CAD build for the part. Positions are in the model's coordinates, mm. A direction names the side the tool comes from. Coordinates: 2 decimals unless noted, no trailing zeros. Loops run counter-clockwise (first coordinate to the right, second up) from the corner with the lowest first, then second, coordinate; pieces in that order, holes last.
1) Saw through at C-C, the plane x = 15.3. Write the cut outline in (y, z).
2) Wall check: line 1 along Y through (x, z) = (0, 2.45); line 2 along Z through (x, y) = (3, 0.5). Give the ranges that are in metal, low to high.
3) Saw through at D-D, the plane y = -1.5. Write the cut outline in (x, z).
4) Saw through at A-A, the plane x = 0. Write the cut outline in (y, z).
5) Pin check, flat tips, straight feed: pin 1 Ø3.5 at (x, y) = (8, -0.5) entering from +Z; pin 2 Ø3 at (y, z) = (-3, 4.5) entering from +X; pin 3 Ø0.7 at (x, y) = (15.3, 0) entering from -Z; pin 4 Ø4 at (x, y) = (0, 0) entering from -Z. Stop position of each tip, or through.
6) Which spindle directions (+Z, -Z, +X, -X, +Y, -Y) get a long thin tool onto all of the face, cutting with end or side? Do faces 1 (the cylindrical face through (18.354, 0.23, 0.986)), 2 (the cylindrical face through (0.509, 2.294, 4.218)), 3 (the flat face through (-1, 1, 2.1)). Say none if no direction does.
7) Saw through at B-B, the plane z = 3.95. Write the cut outline in (x, y).
Autodesk Fusion 360 part; units mm, degrees
sketch "スケッチ1" plane through (0, 0, 0) normal (0, 0, 1) x (1, 0, 0)
  line L0 (2.1071, 3.4) -> (-2.1071, 3.4) construction
  line L1 (-2.1071, -3.4) -> (2.1071, -3.4) construction
  line L2 (22.8, 3.4) -> (-22.8, 3.4) construction
  line L3 (-22.8, 3.4) -> (-22.8, -3.4) construction
  line L4 (-22.8, -3.4) -> (22.8, -3.4) construction
  line L5 (22.8, -3.4) -> (22.8, 3.4) construction
  line L6 (22.8, 3.4) -> (-22.8, -3.4) construction
  line L7 (-22.8, 3.4) -> (22.8, -3.4) construction
  line L8 (-2.1071, 3.4) -> (-20.4231, 2.497)
  line L9 (-2.1071, -3.4) -> (-20.4231, -2.497)
  line L10 (2.1071, 3.4) -> (20.4231, 2.497)
  line L11 (2.1071, -3.4) -> (20.4231, -2.497)
  arc A0 (-20.4231, 2.497) -> (-20.4231, -2.497) centre (-20.3, 0) ccw
  arc A1 (20.4231, -2.497) -> (20.4231, 2.497) centre (20.3, 0) ccw
  arc A2 (2.1071, 3.4) -> (-2.1071, 3.4) centre (0, 0) ccw
  arc A3 (-2.1071, 3.4) -> (-2.1071, -3.4) centre (0, 0) ccw
  arc A4 (2.1071, -3.4) -> (2.1071, 3.4) centre (0, 0) ccw
  arc A5 (-2.1071, -3.4) -> (2.1071, -3.4) centre (0, 0) ccw
  line L12 (-2.1071, 3.4) -> (2.1071, 3.4)
  line L13 (-2.1071, -3.4) -> (2.1071, -3.4)
  circle A6 centre (-20.3, 0) radius 0.6
  circle A7 centre (-17.8, 0) radius 0.6
  circle A8 centre (-15.3, 0) radius 0.6
  circle A9 centre (-12.8, 0) radius 0.6
  circle A10 centre (-10.3, 0) radius 0.6
  line L14 (0, 1.75) -> (0, 22.5) construction
  circle A11 centre (10.3, 0) radius 0.6
  circle A12 centre (12.8, 0) radius 0.6
  circle A13 centre (15.3, 0) radius 0.6
  circle A14 centre (17.8, 0) radius 0.6
  circle A15 centre (20.3, 0) radius 0.6
  dimension "d1" = 8
  dimension "d5" = 6.8
  dimension "d6" = 45.6
  dimension "d7" = 6.8
  dimension "d8" = 2.5
  dimension "d9" = 2.5
  dimension "d10" = 1.2
  dimension "d11" = 2.5
  dimension "d14" = 2.5
  dimension "d15" = 0
  dimension "d16" = 10
extrude "押し出し1" add sketch "スケッチ1" along normal blind 5.5 contours A3 A4 L12 L13 | A2 L12 | A5 L13 makes body 1
extrude "押し出し2" add sketch "スケッチ1" along normal blind 2 contours L8 L9 A0 A3 | L10 L11 A1 A4 bodies 1
sketch "スケッチ2" plane through (0, 0, 5.5) normal (0, 0, 1) x (-1, 0, 0)
  circle A0 centre (0, 0) radius 4
  circle A1 centre (0, 0) radius 1
  circle A2 centre (0, 0) radius 2.35
  dimension "d23" = 2
  dimension "d24" = 4.7
extrude "押し出し3" cut sketch "スケッチ2" against normal through all contours A1 bodies 1
extrude "押し出し4" cut sketch "スケッチ2" against normal blind 2.6 contours A2 bodies 1
sketch "スケッチ3" plane through (0, 0, 0) normal (0, 0, 1) x (1, 0, 0)
  circle A0 centre (0, 0) radius 3.1
  dimension "d28" = 6.2
extrude "押し出し5" cut sketch "スケッチ3" along normal blind 2.1 bodies 1
copy_body "ボディ -> コンポーネント1" bodies 1 removing the originals makes body 2 in component "Component'"
component "Component'" placed x (1, 0, 0) y (0, 1, 0) z (0, 0, 1) at (0, 0, 0)
Data:
1. outline: (-2.75, 0) - (-0.6, 0) - (-0.6, 2) - (-2.75, 2) - close; (0.6, 0) - (2.75, 0) - (2.75, 2) - (0.6, 2) - close
2. line 1: y = -4 to -1, 1 to 4
2. line 2: z = 2.1 to 5.5
3. outline: (-22.3, 0) - (-2.71, 0) - (-2.71, 2.1) - (2.71, 2.1) - (2.71, 0) - (22.3, 0) - (22.3, 2) - (3.71, 2) - (3.71, 5.5) - (1.81, 5.5) - (1.81, 2.9) - (-1.81, 2.9) - (-1.81, 5.5) - (-3.71, 5.5) - (-3.71, 2) - (-22.3, 2) - close
4. outline: (-4, 0) - (-3.1, 0) - (-3.1, 2.1) - (-1, 2.1) - (-1, 2.9) - (-2.35, 2.9) - (-2.35, 5.5) - (-4, 5.5) - close; (1, 2.1) - (3.1, 2.1) - (3.1, 0) - (4, 0) - (4, 5.5) - (2.35, 5.5) - (2.35, 2.9) - (1, 2.9) - close
5. pin 1: stops at z = 2
5. pin 2: stops at x = 3.71
5. pin 3: passes through
5. pin 4: stops at z = 2.1
6. face 1: +Z, -Z
6. face 2: +Z
6. face 3: -Z
7. outline: circle Ø8 at (0, 0); hole circle Ø4.7 at (0, 0)
